from build123d import *

# Parameters (mm, degrees)
F0_W           = 138.9888
F0_H           = 419.989
F1_DEPTH       = 12.7
F3_D           = 8.8
F3_CBORE_D     = 14.25
F3_CBORE_DEPTH = 8
F4_W           = 419.989
F4_H           = 12.7
F5_DEPTH       = 12.7


# Not quite as in the source:
# - a feature names something its author has since deleted; it is built from what else it names


with BuildPart() as f1:
    # F0 (on Top) → F1 (new body)
    with BuildSketch(Plane.XY):
        with Locations((69.4944, 309.9943)):
            Rectangle(F0_W, F0_H)
    extrude(amount=F1_DEPTH)

    # F3 (through all)
    with Locations(Plane.XY.offset(12.7)):
        with Locations((83.9978, 465.0339696), (83.9978, 385.0339772), (83.9978, 305.0339848), (83.9978, 225.0339924), (83.9978, 145.034), (108.9914, 130.0226), (108.9914, 180.0225), (108.9914, 230.0224), (108.9914, 280.0223), (108.9914, 330.0222), (108.9914, 380.0221), (108.9914, 430.022), (108.9914, 480.0219)):
            CounterBoreHole(F3_D / 2, F3_CBORE_D / 2, F3_CBORE_DEPTH)

    # F4 (on face) → F5 (join)
    with BuildSketch(Plane.YZ.offset(138.9888)):
        with Locations((309.9943, 6.35)):
            Rectangle(F4_W, F4_H)
    extrude(amount=F5_DEPTH)


solid = f1.part
Verification items for the finished model (mm, model axes). A direction names the side the tool comes from. Coordinates: 2 decimals unless noted, no trailing zeros. Put each result on its own line as item: value. Start each with the question number.
1. Cross-section at A-A, the plane z = 10.75. Count the separate pieces of the cut face and the enclosed holes in it, then the cut area to 3 significant figures.
2. Go/stop test with a flat-tipped pin: pin 1 Ø11.5 at (x, y) = (83, 304.5) entering from +Z. Record where the tip stops, or that it passes through.
3. Mould release check, pull along Y, two halves, no side actions. Record for faces 1 (the flat face through (0, 307, 6)), 2 (the cylindrical face through (112.82, 136.03, 8.76)): released by +Y, released by -Y, zero draft, split by the parting line, or undercut.
4. Access from +Z, -Z, +X, -X, +Y, -Y to the whole of each face (thin tool, end or side, straight path). Record for faces 3 (the cylindrical face through (88.394, 145.227, 2.317)), 4 (the cylindrical face through (115.79, 232.16, 8.76)).
5. Material ranges on L1, parallel to Y at x = 84, z = 9; L2, parallel to X at y = 305, z = 4.75; L3, parallel to X at y = 229.5, z = 4, recorded low to high. Write a range as [from, to].
Computed:
1. separate pieces: 1
1. enclosed holes: 13
1. area: 61,600 mm2
2. pin 1: z = 4.7
3. face 1: zero draft
3. face 2: undercut
4. face 3: +Z, -Z
4. face 4: +Z
5. L1: [100, 137.91], [152.16, 217.91], [232.16, 297.91], [312.16, 377.91], [392.16, 457.91], [472.16, 519.99]
5. L2: [0, 76.87], [91.12, 151.69]
5. L3: [0, 104.62], [113.36, 151.69]
